Build history of the part. All positions in model axes, mm. A direction names the side the tool comes from. Round coordinates to 2 decimals unless told otherwise and drop trailing zeros. Order: outer loops, then holes, each group sorted by start corner. A loop starts at its lowest first (then second) coordinate and runs counter-clockwise, first axis right, second up. Notation, with made-up numbers: M 77.25,8.5 L 92.25,8.5 A3 cw 92.25,12.5 Z; hole C 15,81.25 d1. An arc over 180 degrees is marked long. One line per item, written item: value. Start each with the question number.
Item 1: Probe L1, parallel to X at y = 27, z = 16; L2, parallel to Y at x = -16, z = 5.25; L3, parallel to Z at x = -8, y = -1. List the from-to ranges inside material, lowest first.
Item 2: Pin check, flat tips, straight feed: pin 1 (4 mm diameter, centred on y = 15.5, z = 8.5, fed in from +X); pin 2 (3 mm diameter, centred on x = -9, z = 15.5, fed in from +Y); pin 3 (1 mm diameter, centred on x = -18.5, y = 16, fed in from -Z). Stop position of each tip, or through.
Item 3: Band-saw the part on D-D, the plane y = 27. Write the cut outline in (x, z).
Item 4: Band-saw the part on C-C, the plane x = -9. Write the cut outline in (y, z).
Item 5: Tool access for faces 4 (the flat face through (-5.16, 9.01, 17.8)), 5 (the flat face through (-5.16, 9.01, 1.25)), 6 (the flat face through (-19.286, 24, 9)): list every direction of +Z, -Z, +X, -X, +Y, -Y with a clear straight run to the whole face (end or side of a thin tool).
Item 6: Band-saw the part on A-A, the plane z = 11.5. Write the cut outline in (x, y).
Item 7: Band-saw the part on B-B, the plane y = -5. Write the cut outline in (x, z) (3 decimals).
Item 8: Two-plate mould, pull along Z, no slides. Class faces 1 (the cylindrical face through (-0.48, 0.64, 3.89)), 2 (the flat face through (-37.048, 15.036, 17.798)), 3 (the flat face through (-20.574, 24.108, 1.252)): +Z half, -Z half, draft (parallel to the pull), parting line (faces both ways), or undercut.
```python
from build123d import *

# Parameters (mm, degrees)
F1_DEPTH = 19.05
F2_SIZE  = 2.54
F4_D     = 12.7


with BuildPart() as f1:
    # F0 (on Top) → F1 (new body)
    with BuildSketch(Plane.XY):
        Polygon((-19.2860513926, 35.6976958707), (-38.3360513926, 35.6976958707), (-38.3360513926, -8.7523041293), (6.1139486074, -8.7523041293), (6.1139486074, 10.2976958707), (-19.2860513926, 10.2976958707), align=None)
    extrude(amount=F1_DEPTH)

    # F2
    f2_edges = [f1.edges().sort_by_distance(p)[0] for p in [
        (-19.286051, 10.297696, 9.525),
        (-28.811051, 35.697696, 19.05),
        (-38.336051, 13.472696, 19.05),
        (-16.111051, -8.752304, 19.05),
        (-38.336051, 13.472696, 0),
        (-38.336051, -8.752304, 9.525),
        (-16.111051, -8.752304, 0),
        (-6.586051, 10.297696, 0),
        (-6.586051, 10.297696, 19.05),
        (-19.286051, 22.997696, 0),
        (-19.286051, 22.997696, 19.05),
    ]]
    chamfer(f2_edges, length=F2_SIZE)

    # F4 (through all)
    with Locations(Plane(origin=(0, 10.2976958707, 0), x_dir=(-1, 0, 0), z_dir=(0, 1, 0))):
        with Locations((3.4110513926, 9.525)):
            Hole(F4_D / 2)


solid = f1.part
```
Output:
1. L1: x = -38.34 to -19.29
1. L2: y = -8.75 to 10.3
1. L3: z = 0 to 5.14, 13.91 to 19.05
2. pin 1: stops at x = -19.29
2. pin 2: stops at y = 10.3
2. pin 3: passes through
3. outline: M -38.34,2.54 L -35.8,0 L -21.83,0 L -19.29,2.54 L -19.29,16.51 L -21.83,19.05 L -35.8,19.05 L -38.34,16.51 Z
4. outline: M -8.75,2.54 L -6.21,0 L 7.76,0 L 10.3,2.54 L 10.3,6.51 L -8.75,6.51 Z; M -8.75,12.54 L 10.3,12.54 L 10.3,16.51 L 7.76,19.05 L -6.21,19.05 L -8.75,16.51 Z
5. face 4: +Z, +X, +Y
5. face 5: -Z, +X, +Y
5. face 6: +Z, -Z, +X, +Y
6. outline: M -38.34,-6.21 L -35.8,-8.75 L -9.45,-8.75 L -9.45,10.3 L -16.75,10.3 L -19.29,12.84 L -19.29,35.7 L -38.34,35.7 Z; M 2.62,-8.75 L 6.11,-8.75 L 6.11,10.3 L 2.62,10.3 Z
7. outline: M -38.336,2.54 L -35.796,0 L 6.114,0 L 6.114,19.05 L -35.796,19.05 L -38.336,16.51 Z; hole C -3.411,9.525 d12.7
8. face 1: undercut
8. face 2: +Z half
8. face 3: -Z half
